Geometry check sheet. Reference: the model listing, model coordinates, mm. Give positions to 0.01 mm unless a question says otherwise; leave off trailing zeros. Loops run counter-clockwise (first coordinate to the right, second up) from the corner with the lowest first, then second, coordinate; pieces in that order, holes last. Notation, with made-up numbers: (12.25, -20) -> (64.25, -20) arc R13 ccw to (64.25, -16) -> close; hole circle Ø11 at (22.5, 40.5). An arc over 180 degrees is marked (long way). Answer as a JSON object with one key per item and string values.
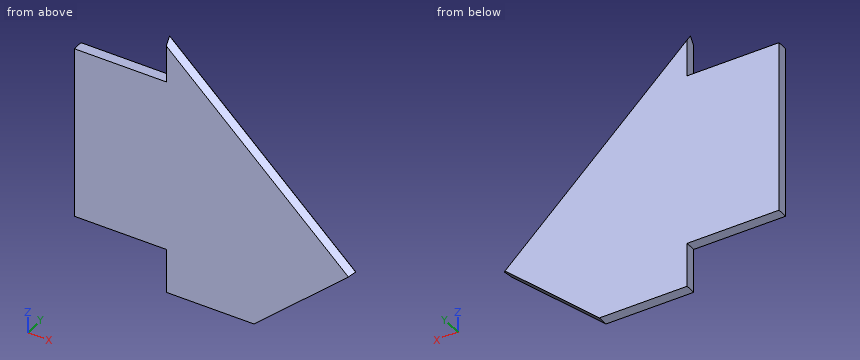
Solid Edge part; units mm, degrees
sketch "Sketch1" plane through (0, 0, 0) normal (0, -1, 0) x (1, 0, 0)
  line L0 (55.5, 25) -> (2.5, 75)
  line L1 (2.5, 62.3) -> (2.5, 75)
  line L2 (0, 62.3) -> (2.5, 62.3)
  line L3 (0, 12.7) -> (0, 62.3)
  line L4 (0, 12.7) -> (2.5, 12.7)
  line L5 (2.5, 12.7) -> (2.5, 0)
  line L6 (2.5, 0) -> (27.5, 0)
  line L7 (27.5, 0) -> (55.5, 25)
extrude "Protrusion1" add sketch "Sketch1" along normal mid plane 3
chamfer "Chamfer_1" distance 1.5 angle 45 2 edges at (29, -1.5, 50) (29, 1.5, 50)
sketch "Sketch2" plane through (27.1885, -1.5, 36.4689) normal (0, -1, 0) x (-1, 0, 0)
  line L0 (24.6885, -25.8311) -> (50.8759, -25.8311)
  line L1 (50.8759, -25.8311) -> (50.8759, 23.7689)
  line L2 (50.8759, 23.7689) -> (24.6885, 23.7689)
  line L3 (24.6885, 23.7689) -> (24.6885, -25.8311)
extrude "Protrusion2" add sketch "Sketch2" against normal up to vertex (3 mm away)
1) Section check A-A on y = -0.7. Record the cut outline in (x, z), plus the area to 3 significant figures.
Geometry check:
{"outline": "(-23.69, 12.7) -> (2.5, 12.7) -> (2.5, 0) -> (27.5, 0) -> (54.98, 24.53) -> (2.5, 74.04) -> (2.5, 62.3) -> (-23.69, 62.3) -> close", "area": "3,550 mm2"}
2) Material ranges on line 1 along Z through (x, y) = (-4.5, -0.15); line 2 along X through (y, z) = (-0.25, 17); line 3 along X through (y, z) = (-1.25, 12), recorded low to high. Write a range as from..to.
Geometry check:
{"line 1": "z = 12.7..62.3", "line 2": "x = -23.69..46.54", "line 3": "x = 2.5..40.94"}
3) Section check B-B on x = -7. Record the cut outline in (y, z).
Geometry check:
{"outline": "(-1.5, 12.7) -> (1.5, 12.7) -> (1.5, 62.3) -> (-1.5, 62.3) -> close"}
4) Section check C-C on z = 19.5. Record the cut outline in (x, y).
Geometry check:
{"outline": "(-23.69, -1.5) -> (49.34, -1.5) -> (49.34, 1.5) -> (-23.69, 1.5) -> close"}
